```python
from build123d import *

# Parameters (mm, degrees)
F1_DEPTH = 12
F2_R     = 0.99999
F3_R     = 2.99999


# Not quite as in the source:
# - a fillet or chamfer is up to 0.001 mm smaller than in the source, because OpenCascade refuses the exact size


with BuildPart() as f1:
    # F0 (on Top) → F1 (new body)
    with BuildSketch(Plane.XY):
        Polygon((23.3803613689, 1.1605409955), (5.8803613689, 1.1605409955), (5.8803613689, -1.8394590045), (26.3803613689, -1.8394590045), (26.3803613689, -0.8394590045), (38.3803613689, -0.8394590045), (38.3803613689, -1.8394590045), (58.8803613689, -1.8394590045), (58.8803613689, 1.1605409955), (41.3803613689, 1.1605409955), align=None)
    extrude(amount=F1_DEPTH)

    # F2 (radius 1 in the source; OpenCascade refuses exactly that, so slightly less here)
    f2_edges = [f1.edges().sort_by_distance(p)[0] for p in [
        (38.380361, -0.839459, 6),
        (26.380361, -0.839459, 6),
    ]]
    fillet(f2_edges, radius=F2_R)

    # F3 (radius 3 in the source; OpenCascade refuses exactly that, so slightly less here)
    f3_edges = [f1.edges().sort_by_distance(p)[0] for p in [
        (5.880361, 1.160541, 6),
        (58.880361, 1.160541, 6),
    ]]
    fillet(f3_edges, radius=F3_R)


solid = f1.part
```
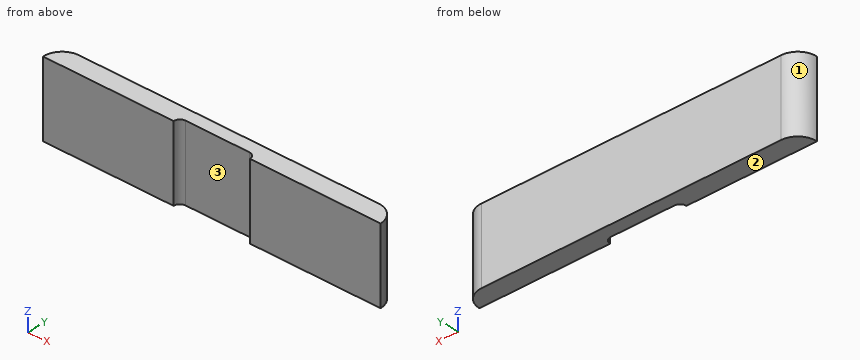
Here's how the part is built. I have some questions about the finished solid (model axes, mm). Face numbers are marked on the shaded views. Coordinates: 2 decimals unless noted, no trailing zeros. Order: outer loops, then holes, each group sorted by start corner. A loop starts at its lowest first (then second) coordinate and runs counter-clockwise, first axis right, second up. Notation, with made-up numbers: (58, 57.25) - (68, 57.25) arc R30 cw to (68, 93.25) - close; hole circle Ø5 at (54, -4.75). An arc over 180 degrees is marked (long way). One line per question, with ' | ' between items.
(1) If we mould it in two halves opening along X, with no side actions, what happens to the marked faces 1, 2 and 3? For each: pulls with the +X half, pulls with the -X half, needs draft (parallel to the pull), parting line crosses it, or undercut.
Report:
face 1: pulls with the -X half | face 2: needs draft | face 3: undercut
(2) Will this pin go through, and if not, where does the flat tip stop? pin 1 (3 mm diameter, centred on x = 31.5, z = 4, fed in from -Y).
Report:
pin 1: stops at y = -0.84
(3) Suppose I cut it at C-C on y = -0.25. List the corners of the cut face in (x, z) for me.
Report:
outline: (6.34, 0) - (58.42, 0) - (58.42, 12) - (6.34, 12) - close
(4) Suppose I cut it at B-B on x = 35.5. List the corners of the cut face in (y, z) for me, and give its area (3 significant figures).
Report:
outline: (-0.84, 0) - (1.16, 0) - (1.16, 12) - (-0.84, 12) - close | area: 24.0 mm2
(5) If I drill on L1, parallel to X at y = -1.15, z = 3.25; L2, parallel to Y at x = 35, z = 4.5; L3, parallel to X at y = -1.2, z = 5.25, over which ranges is the centre line in solid material (lowest first)?
Report:
L1: x = 5.96 to 26.66, 38.1 to 58.8 | L2: y = -0.84 to 1.16 | L3: x = 5.95 to 26.61, 38.15 to 58.81
